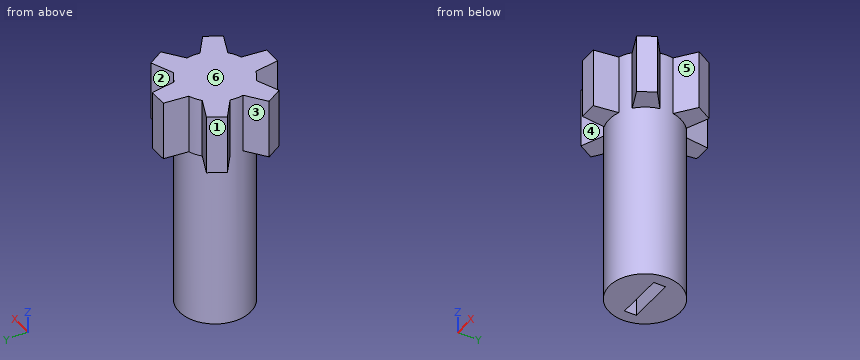
```python
from build123d import *

# Parameters (mm, degrees)
ESQUISSE1_R                  = 3
MAIN_EXTRUSION_DEPTH         = 5
GEAR_ELEMENT_DEPTH           = 5
R_P_TITION_CIRCULAIRE1_COUNT = 6
ESQUISSE3_R                  = 3
MAIN_AXE_DEPTH               = 15
ESQUISSE4_W                  = 4
ESQUISSE4_H                  = 1
AXE_TRAIT_DEPTH              = 3


with BuildPart() as part:
    # Esquisse1 → Main Extrusion (new body)
    with BuildSketch(Plane.XY):
        Circle(ESQUISSE1_R)
    extrude(amount=MAIN_EXTRUSION_DEPTH)

    # Esquisse2 → Gear Element (add)
    with BuildSketch(Plane.XY.offset(5)):
        Polygon((-1, 2.828427125), (1, 2.828427125), (0.75, 4.828427125), (-0.75, 4.828427125), align=None)
    gear_element = extrude(amount=-GEAR_ELEMENT_DEPTH)

    # Répétition circulaire1: Gear Element ×6 about axis
    r_p_tition_circulaire1_axis = Axis((0, 0, 0), (0, 0, 1))
    for i in range(1, R_P_TITION_CIRCULAIRE1_COUNT):
        add(gear_element.rotate(r_p_tition_circulaire1_axis, i * 360 / R_P_TITION_CIRCULAIRE1_COUNT))

    # Esquisse3 → Main Axe (add)
    with BuildSketch(Plane(origin=(0, 0, 0), x_dir=(-1, 0, 0), z_dir=(0, 0, -1))):
        Circle(ESQUISSE3_R)
    extrude(amount=MAIN_AXE_DEPTH)

    # Esquisse4 → Axe Trait (cut)
    with BuildSketch(Plane(origin=(0, 0, -15), x_dir=(-1, 0, 0), z_dir=(0, 0, -1))):
        Rectangle(ESQUISSE4_W, ESQUISSE4_H)
    extrude(amount=-AXE_TRAIT_DEPTH, mode=Mode.SUBTRACT)


solid = part.part
```
Can you work these out from the model? Positions are in its coordinate system, mm. Face numbers are marked on the shaded views. A direction names the side the tool comes from. Give positions to 0.01 mm unless a question says otherwise; leave off trailing zeros. Write each loop counter-clockwise with the first axis right and the second up, starting at its lowest first coordinate (ties: lowest second). Pieces come first, ordered by that corner, then holes. Notation, with made-up numbers: (-6.75, 64) - (46.25, 64) arc R23 ccw to (46.25, 80) - close; hole circle Ø4 at (15, 16). An arc over 180 degrees is marked (long way). Write item = value, one per line. Start each with the question number.
1. Imagine slicing it at A-A (x = 3.25). Please give me the cut outline in (y, z).
2. On a 3-axis mill with a long thin cutter (end or side, diameter ignored), from which of +Z, -Z, +X, -X, +Y, -Y can I reach the whole of each face in a straight line? I mean the marked faces 1, 2 and 3. Say none if no direction works.
3. Thinking about a two-plate mould opening in X: for the marked faces 4, 5 and 6, which applies, released by +X, released by -X, zero draft, split by the parting line, or undercut?
4. Imagine slicing it at C-C (y = 0). Please give me the cut outline in (x, z), and give its area (3 significant figures).
5. Imagine slicing it at D-D (z = -6). Please give me the cut outline in (x, y).
6. Please list where these lines run through material, in increasing order: line 1 (Z direction, x = 0.75, y = -0.25); line 2 (Y direction, x = 0, z = -1.5); line 3 (Z direction, x = 0.75, y = 4.5).
7. For pin 1 (1.1 mm diameter, centred on y = 0, z = -14, fed in from -X); pin 2 (2 mm diameter, centred on x = -0.5, y = -4, fed in from -Z); pin 3 (0.8 mm diameter, centred on y = 0, z = -14, fed in from +X); pin 4 (1.3 mm diameter, centred on x = -3, y = -1.5, fed in from -Z), each with a flat end and sliding along its axis, tell me the tip position at first contact or that it passes through.
8. Imagine slicing it at B-B (x = 0). Please give me the cut outline in (y, z), and give its area (3 significant figures).
Worked answers:
q1.outline = (-2.83, 0) - (-0.78, 0) - (-0.78, 5) - (-2.83, 5) - close; (0.78, 0) - (2.83, 0) - (2.83, 5) - (0.78, 5) - close
q2.face_1 = +Z, -Z, -X, +Y
q2.face_2 = +Z, -Z, +Y
q2.face_3 = +Z, -Z, -X
q3.face_4 = undercut
q3.face_5 = released by +X
q3.face_6 = zero draft
q4.outline = (-3, -15) - (-2, -15) - (-2, -12) - (2, -12) - (2, -15) - (3, -15) - (3, 5) - (-3, 5) - close
q4.area = 108 mm2
q5.outline = circle Ø6 at (0, 0)
q6.line_1 = -12 to 5
q6.line_2 = -3 to 3
q6.line_3 = 0 to 5
q7.pin_1 = -3
q7.pin_2 = 0
q7.pin_3 = 3
q7.pin_4 = -15
q8.outline = (-4.83, 0) - (-3, 0) - (-3, -15) - (-0.5, -15) - (-0.5, -12) - (0.5, -12) - (0.5, -15) - (3, -15) - (3, 0) - (4.83, 0) - (4.83, 5) - (-4.83, 5) - close
q8.area = 135 mm2
